from build123d import *

# Parameters (mm, degrees)
SKETCH_2_R          = 1.3
EXTRUDE_2_DEPTH     = 3
SKETCH_4_W          = 2
SKETCH_4_H          = 4
EXTRUDE_3_DEPTH     = 4
SKETCH_6_R          = 1.1
CUT_EXTRUDE_2_DEPTH = 50.25


with BuildPart() as part:
    # 草图2 → 凸台-拉伸2 (new body)
    with BuildSketch(Plane.XY):
        with BuildLine():
            Line((-3.5, -10), (-3.5, 1))
            ThreePointArc((-3.5, 1), (-2.767766953, 2.767766953), (-1, 3.5))
            Line((-1, 3.5), (59, 3.5))
            ThreePointArc((59, 3.5), (60.767766953, 2.767766953), (61.5, 1))
            Line((61.5, 1), (61.5, -10))
            ThreePointArc((61.5, -10), (60.767766953, -11.767766953), (59, -12.5))
            Line((59, -12.5), (-1, -12.5))
            ThreePointArc((-1, -12.5), (-2.767766953, -11.767766953), (-3.5, -10))
        make_face()
        with Locations((58, -4.5)):
            Circle(SKETCH_2_R, mode=Mode.SUBTRACT)
        with Locations((0, -4.5)):
            Circle(SKETCH_2_R, mode=Mode.SUBTRACT)
    extrude(amount=EXTRUDE_2_DEPTH)

    # 草图4 → 凸台-拉伸3 (add)
    with BuildSketch(Plane.XY.offset(3)):
        with Locations((13.25, 1.5)):
            Rectangle(SKETCH_4_W, SKETCH_4_H)
        with Locations((17.75, 1.5)):
            Rectangle(SKETCH_4_W, SKETCH_4_H)
        with Locations((40.25, 1.5)):
            Rectangle(SKETCH_4_W, SKETCH_4_H)
        with Locations((44.75, 1.5)):
            Rectangle(SKETCH_4_W, SKETCH_4_H)
        with Locations((15.75, -10.5)):
            Rectangle(SKETCH_4_W, SKETCH_4_H)
        with Locations((20.25, -10.5)):
            Rectangle(SKETCH_4_W, SKETCH_4_H)
        with Locations((37.75, -10.5)):
            Rectangle(SKETCH_4_W, SKETCH_4_H)
        with Locations((42.25, -10.5)):
            Rectangle(SKETCH_4_W, SKETCH_4_H)
    extrude(amount=EXTRUDE_3_DEPTH)

    # 草图6 → 切除-拉伸2 (cut, through all)
    with BuildSketch(Plane.ZY.offset(-12.25)):
        with Locations((5, 1.5)):
            Circle(SKETCH_6_R)
        with Locations((5, -10.5)):
            Circle(SKETCH_6_R)
    extrude(amount=-CUT_EXTRUDE_2_DEPTH, mode=Mode.SUBTRACT)


solid = part.part
Could you check a few things on this model? Use its own coordinates, in mm. A direction names the side the tool comes from. Coordinates: 2 decimals unless noted, no trailing zeros. Order: outer loops, then holes, each group sorted by start corner. A loop starts at its lowest first (then second) coordinate and runs counter-clockwise, first axis right, second up. Notation, with made-up numbers: (85.5, -3.75) - (131.5, -3.75) arc R7 ccw to (131.5, 0.25) - close; hole circle Ø9 at (69.25, 31). An arc over 180 degrees is marked (long way). Answer in a Markdown table with one row per item. Add a question column.
(1) On a 3-axis mill with a long thin cutter (end or side, diameter ignored), from which of +Z, -Z, +X, -X, +Y, -Y can I reach the whole of each face in a straight line? I mean faces 1 (the face through (12.25, 2.4, 4.1)), 2 (the face through (21.25, -9.6, 4.1)), 3 (the face through (42, -8.5, 5)). Say none if no direction works.
(2) I need wall thicknesses on L1, parallel to X at y = -10.5, z = 3.25; L2, parallel to Y at x = 37.9, z = 5; L3, parallel to Y at x = 12.9, z = 5. Which ranges of each line are inside material? Lowest first, please.
(3) If we section it at D-D, the plane x = 18: Please give me the cut outline in (y, z).
(4) If we section it at B-B, the plane z = 2: Please give me the cut outline in (x, y), then the cut area to 3 significant figures.
(5) If we mould it in two halves opening along Y, with no side actions, what happens to faces 4 (the face through (13, 2, 7)), 5 (the face through (-2.787, 2.748, 1.479)), 6 (the face through (13.236, 2.243, 4.189))? For each: released by +Y, released by -Y, zero draft, split by the parting line, or undercut.
(6) If we section it at C-C, the plane x = 0: Please give me the cut outline in (y, z), then the cut area to 3 significant figures.
(7) Will these pins go through, and if not, where does the flat tip stop? pin 1 (1.2 mm diameter, centred on y = 1, z = 5.5, fed in from -X); pin 2 (1.2 mm diameter, centred on y = 2, z = 4.5, fed in from +X); pin 3 (2 mm diameter, centred on x = 38, z = 4.5, fed in from +Y).
(8) If we section it at A-A, the plane y = -4.5: Please give me the cut outline in (x, z).
Results are:
| question | item | result |
|---|---|---|
| 1 | face 1 | +Z, -X, +Y, -Y |
| 1 | face 2 | +Z, +Y, -Y |
| 1 | face 3 | +Z, +X, -X, +Y |
| 2 | L1 | x = 14.75 to 16.75, 19.25 to 21.25, 36.75 to 38.75, 41.25 to 43.25 |
| 2 | L2 | y = -12.5 to -11.6, -9.4 to -8.5 |
| 2 | L3 | y = -0.5 to 0.4, 2.6 to 3.5 |
| 3 | outline | (-12.5, 0) - (3.5, 0) - (3.5, 7) - (-0.5, 7) - (-0.5, 3) - (-12.5, 3) - close; hole circle Ø2.2 at (1.5, 5) |
| 4 | outline | (-3.5, -10) arc R2.5 ccw to (-1, -12.5) - (59, -12.5) arc R2.5 ccw to (61.5, -10) - (61.5, 1) arc R2.5 ccw to (59, 3.5) - (-1, 3.5) arc R2.5 ccw to (-3.5, 1) - close; hole circle Ø2.6 at (0, -4.5); hole circle Ø2.6 at (58, -4.5) |
| 4 | area | 1,020 mm2 |
| 5 | face 4 | zero draft |
| 5 | face 5 | released by +Y |
| 5 | face 6 | undercut |
| 6 | outline | (-12.5, 0) - (-5.8, 0) - (-5.8, 3) - (-12.5, 3) - close; (-3.2, 0) - (3.5, 0) - (3.5, 3) - (-3.2, 3) - close |
| 6 | area | 40.2 mm2 |
| 7 | pin 1 | stops at x = 12.25 |
| 7 | pin 2 | stops at x = 45.75 |
| 7 | pin 3 | stops at y = -8.5 |
| 8 | outline | (-3.5, 0) - (-1.3, 0) - (-1.3, 3) - (-3.5, 3) - close; (1.3, 0) - (56.7, 0) - (56.7, 3) - (1.3, 3) - close; (59.3, 0) - (61.5, 0) - (61.5, 3) - (59.3, 3) - close |
